Autodesk Inventor part; units mm, degrees
ref_plane "YZ Plane" through (0, 0, 0) normal (1, 0, 0) x (0, 1, 0)
ref_plane "XZ Plane" through (0, 0, 0) normal (0, 1, 0) x (-1, 0, 0)
ref_plane "XY Plane" through (0, 0, 0) normal (0, 0, 1) x (1, 0, 0)
sketch "Sketch1" plane through (0, 0, 0) normal (0, 0, 1) x (1, 0, 0)
  line L0 (0, 0) -> (50, 0)
  line L1 (50, 0) -> (50, 125)
  line L2 (50, 125) -> (0, 125)
  line L3 (0, 125) -> (0, 0)
  dimension "d0" = 50
  dimension "d1" = 125
extrude "Extrusion1" add sketch "Sketch1" along normal blind 15
sketch "Sketch2" plane through (0, 0, 15) normal (0, 0, 1) x (1, 0, 0)
  point P0 (25, 25)
hole "Hole1" at (25, 25, 15) direction (0, 0, -1) diameter 20 end through all
sketch "Sketch3" plane through (0, 0, 15) normal (0, 0, 1) x (1, 0, 0)
  circle A0 centre (25, 25) radius 10
  circle A1 centre (25, 25) radius 12.5
  dimension "d11" = 25
extrude "Extrusion2" add sketch "Sketch3" along normal blind 7.5
sketch "Sketch4" plane through (0, 0, 0) normal (0, -1, 0) x (1, 0, 0)
  line L0 (50, 0) -> (50, 15)
  line L1 (50, 15) -> (0, 15)
  point P0 (12.5, 7.5)
  point P1 (25, 7.5)
  point P2 (37.5, 7.5)
  dimension "d14" = 12.5
  dimension "d15" = 12.5
  dimension "d16" = 12.5
  dimension "d152" = 7.5
  dimension "d153" = 7.5
  dimension "d154" = 7.5
hole "Hole2" at (12.5, 0, 7.5) at (25, 0, 7.5) at (37.5, 0, 7.5) direction (0, 1, 0) diameter 4.917 depth 10 tip angle 118
sketch "Sketch10" plane through (50, 0, 0) normal (1, 0, 0) x (0, 0, -1)
  line L0 (-15, 125) -> (-15, 0)
  line L1 (0, 0) -> (-15, 0)
  line L2 (0, 125) -> (-15, 125)
  point P0 (-7.5, 25)
  point P1 (-7.5, 50)
  point P2 (-7.5, 95)
  dimension "d112" = 7.5
  dimension "d113" = 25
  dimension "d114" = 25
  dimension "d118" = 30
  dimension "d150" = 7.5
hole "Hole8" at (50, 25, 7.5) at (50, 50, 7.5) at (50, 95, 7.5) direction (-1, 0, 0) diameter 4.917 depth 8 tip angle 118
sketch "Sketch11" plane through (0, 0, 0) normal (-1, 0, 0) x (0, 0, 1)
  circle A0 centre (7.5, 25) radius 2.4585
  line L0 (0, 125) -> (15, 125)
  line L1 (0, 0) -> (15, 0)
  line L2 (15, 0) -> (15, 125)
  point P0 (7.5, 50)
  point P1 (7.5, 95)
  dimension "d119" = 25
  dimension "d120" = 25
  dimension "d121" = 30
  dimension "d151" = 7.5
hole "Hole9" at (0, 25, 7.5) at (0, 50, 7.5) at (0, 95, 7.5) direction (1, 0, 0) diameter 4.917 depth 8 tip angle 118
sketch "Skizze12" plane through (0, 0, 0) normal (0, 0, -1) x (-1, 0, 0)
  line L0 (-50, 0) -> (-50, 125)
  line L1 (-50, 125) -> (0, 125)
  arc A0 (-17.5, 98) -> (-32.5, 98) centre (-25, 98) ccw
  arc A1 (-32.5, 88) -> (-17.5, 88) centre (-25, 88) ccw
  line L2 (-32.5, 88) -> (-32.5, 98)
  line L3 (-17.5, 98) -> (-17.5, 88)
  arc A2 (-36.1, 88) -> (-13.9, 88) centre (-25, 88) ccw
  line L4 (-36.1, 88) -> (-36.1, 98)
  line L5 (-13.9, 98) -> (-13.9, 88)
  arc A3 (-13.9, 98) -> (-36.1, 98) centre (-25, 98) ccw
  point P0 (-45, 115)
  point P1 (-50, 110)
  point P2 (-5, 115)
  point P3 (0, 125)
  point P4 (-25, 93)
  dimension "d80" = 15
  dimension "d81" = 25
  dimension "d82" = 27
  dimension "d83" = 15
  dimension "d84" = 10
  dimension "d86" = 22.2
extrude "Extrusion5" cut sketch "Skizze12" against normal blind 17 contours L3 A1 L2 A0
extrude "Extrusion6" cut sketch "Skizze12" against normal blind 2
sketch "Skizze13" plane through (0, 0, 15) normal (0, 0, 1) x (1, 0, 0)
  arc A0 (32.5, 98) -> (17.5, 98) centre (25, 98) ccw
  arc A1 (11.25, 113.5) -> (7.75, 113.5) centre (9.5, 113.5) ccw
  arc A2 (7.75, 103.5) -> (11.25, 103.5) centre (9.5, 103.5) ccw
  arc A3 (14.5, 113.5) -> (4.5, 113.5) centre (9.5, 113.5) ccw
  arc A4 (4.5, 103.5) -> (14.5, 103.5) centre (9.5, 103.5) ccw
  line L0 (4.5, 103.5) -> (4.5, 113.5)
  line L1 (14.5, 103.5) -> (14.5, 113.5)
  line L2 (7.75, 103.5) -> (7.75, 113.5)
  line L3 (11.25, 103.5) -> (11.25, 113.5)
  dimension "d95" = 3.5
  dimension "d96" = 3.5
  dimension "d97" = 10
  dimension "d98" = 15.5
  dimension "d99" = 10
  dimension "d100" = 10
  dimension "d111" = 15.5
extrude "Extrusion7" cut sketch "Skizze13" against normal blind 17 contours L3 A2 L2 A1
extrude "Extrusion8" cut sketch "Skizze13" against normal blind 10
pattern_linear "Rechteckige Anordnung1" count 2 spacing 31 along (0, -1, 0) count 2 spacing 31 along (1, 0, 0) of "Extrusion8", "Extrusion7"
sketch "Skizze14" plane through (0, 125, 0) normal (0, 1, 0) x (1, 0, 0)
  line L0 (50, 0) -> (50, -15)
  line L1 (0, -15) -> (50, -15)
  point P0 (25, -7.5)
  dimension "d124" = 25
  dimension "d155" = 7.5
hole "Bohrung10" at (25, 125, 7.5) direction (0, -1, 0) diameter 4.917 depth 12 tip angle 118
sketch "Skizze15" plane through (0, 0, 15) normal (0, 0, 1) x (1, 0, 0)
  arc A0 (32.5, 98) -> (17.5, 98) centre (25, 98) ccw
  point P0 (9.5, 91)
  point P1 (40.5, 91)
  point P2 (25, 73.5)
  point P3 (35, 53.5)
  point P4 (15, 53.5)
  dimension "d132" = 17.5
  dimension "d133" = 17.5
  dimension "d134" = 7
  dimension "d159" = 20
  dimension "d160" = 10
  dimension "d161" = 10
  dimension "d162" = 20
hole "Bohrung11" at (9.5, 91, 15) at (40.5, 91, 15) at (25, 73.5, 15) at (35, 53.5, 15) at (15, 53.5, 15) direction (0, 0, -1) diameter 3.242 end through all
sketch "Skizze16" plane through (0, 0, 15) normal (0, 0, 1) x (1, 0, 0)
  arc A0 (17.5, 88) -> (32.5, 88) centre (25, 88) ccw
  point P0 (25, 63)
  dimension "d142" = 25
hole "Bohrung12" at (25, 63, 15) direction (0, 0, -1) diameter 6 end through all
sketch "Skizze17" plane through (0, 0, 15) normal (0, 0, 1) x (1, 0, 0)
  circle A0 centre (25, 25) radius 12.5
  circle A1 centre (25, 25) radius 14.5
  dimension "d163" = 29
extrude "Extrusion9" add sketch "Skizze17" along normal blind 0.5
hole "Bohrung13" at (25, 93, 0) direction (0, 0, 1) diameter 19 end through all
equation "\"d83\" = d80"
equation "\"d96\" = d95"
equation "\"d100\" = d99"
properties part number "lower_part_01"
The model under review builds one solid part; all positions refer to its coordinate system, in mm. A direction names the side the tool comes from. Round coordinates to 2 decimals unless told otherwise and drop trailing zeros. Order: outer loops, then holes, each group sorted by start corner. A loop starts at its lowest first (then second) coordinate and runs counter-clockwise, first axis right, second up.
(1) Mouldability with a two-part tool opening along X and no side actions: class faces 5 (the face through (14.5, 77, 10)), 6 (the face through (15.08, 32.606, 18.951)), 7 (the face through (25, 125, 4)) as released by +X, released by -X, zero draft, split by the parting line, or undercut.
Working result:
face 5: undercut
face 6: split by the parting line
face 7: zero draft
(2) Take a section at A-A, the plane y = 63. State the section outline as (x, z) points.
Working result:
outline: (0, 0) - (22, 0) - (22, 15) - (0, 15) - close; (28, 0) - (50, 0) - (50, 15) - (28, 15) - close
(3) Wall thickness on L1, parallel to X at y = 53.5, z = 12; L2, parallel to Z at x = 46.25, y = 50; L3, parallel to X at y = 63, z = 8.75: over which ranges is each line inside the solid? List them lowest first.
Working result:
L1: x = 0 to 13.38, 16.62 to 33.38, 36.62 to 50
L2: z = 0 to 5.04, 9.96 to 15
L3: x = 0 to 22, 28 to 50
(4) Take a section at D-D, the plane y = 100.5. State the section outline as (x, z) points, plus the area to 3 significant figures.
Working result:
outline: (0, 0) - (14.19, 0) - (14.19, 2) - (17.93, 2) - (17.93, 15) - (13.5, 15) - (13.5, 5) - (5.5, 5) - (5.5, 15) - (0, 15) - close; (32.07, 2) - (35.81, 2) - (35.81, 0) - (50, 0) - (50, 15) - (44.5, 15) - (44.5, 5) - (36.5, 5) - (36.5, 15) - (32.07, 15) - close
area: 363 mm2
(5) For P1, Ø4, axis at y = 50, z = 7.5, coming from the +X side; P2, Ø2, axis at x = 20.5, y = 87, coming from the -Z side; P3, Ø8, axis at x = 8, y = 79.5, coming from the +Z side; P4, Ø3, axis at y = 50, z = 7.5, coming from the +X side, all flat-tipped, find the tip position at first contact; note any pin that passes through.
Working result:
P1: stops at x = 41.72
P2: passes through
P3: stops at z = 15
P4: stops at x = 41.42
(6) Take a section at C-C, the plane z = 6.25. Count the separate pieces of the cut face and the enclosed holes in it, plus the area to 3 significant figures.
Working result:
separate pieces: 1
enclosed holes: 12
area: 4,390 mm2
(7) Tool access review of faces 1 (the face through (4.06, 97.4, 6.97)), 2 (the face through (40.46, 70.75, 2.54)), 3 (the face through (25.94, 5.07, 5.23)), 4 (the face through (40.4, 98.5, 10.1)): name each direction out of +Z, -Z, +X, -X, +Y, -Y from which nothing blocks a thin tool from reaching the whole face with its end or side.
Working result:
face 1: -X
face 2: +Z, -Z
face 3: -Y
face 4: +Z
(8) Take a section at B-B, the plane y = 30.5. State the section outline as (x, z) points.
Working result:
outline: (0, 0) - (16.65, 0) - (16.65, 22.5) - (13.78, 22.5) - (13.78, 15.5) - (11.58, 15.5) - (11.58, 15) - (0, 15) - close; (33.35, 0) - (50, 0) - (50, 15) - (38.42, 15) - (38.42, 15.5) - (36.22, 15.5) - (36.22, 22.5) - (33.35, 22.5) - close
